Build history of the part. All positions in model axes, mm. Face numbers are marked on the shaded views. A direction names the side the tool comes from. Round coordinates to 2 decimals unless told otherwise and drop trailing zeros. Write each loop counter-clockwise with the first axis right and the second up, starting at its lowest first coordinate (ties: lowest second). Pieces come first, ordered by that corner, then holes.
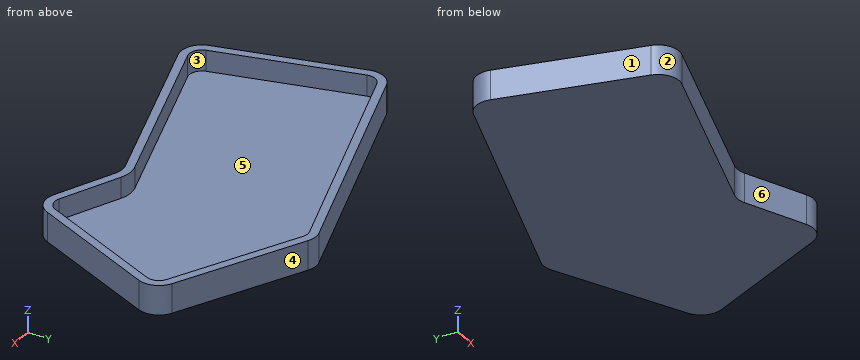
from build123d import *

# Parameters (mm, degrees)
F1_DEPTH = 20
F2_DEPTH = 50
F3_T     = -20


with BuildPart() as f1:
    # F0 (on Top) → F1 (new body)
    with BuildSketch(Plane.XY):
        with BuildLine():
            Line((126.4149565512, 318.7475000366), (-450.1034598535, 122.5814987763))
            ThreePointArc((-450.1034598535, 122.5814987763), (-478.0910883888, 98.8207080739), (-482.3054199281, 62.3498712928))
            Line((-482.3054199281, 62.3498712928), (-393.9558391633, -268.5866574495))
            ThreePointArc((-393.9558391633, -268.5866574495), (-369.4207710673, -299.6767597656), (-329.9698834283, -303.1683916176))
            Line((-329.9698834283, -303.1683916176), (106.3450430495, -159.0930914556))
            ThreePointArc((106.3450430495, -159.0930914556), (124.3346881302, -156.625037143), (142.0194350117, -160.7443028487))
            Line((142.0194350117, -160.7443028487), (282.7517397768, -222.1523142062))
            ThreePointArc((282.7517397768, -222.1523142062), (320.9333231451, -222.9008478399), (348.5065336168, -196.4790448091))
            Line((348.5065336168, -196.4790448091), (481.7955905074, 106.1445162961))
            ThreePointArc((481.7955905074, 106.1445162961), (483.0336988414, 143.3672853444), (458.1969646809, 171.1198362923))
            Line((458.1969646809, 171.1198362923), (164.6807282631, 316.2339391714))
            ThreePointArc((164.6807282631, 316.2339391714), (145.7983966372, 321.3050895289), (126.4149565512, 318.7475000366))
        make_face()
    extrude(amount=F1_DEPTH)

    # F2 (add): a face of the model
    f2_faces = [f1.faces().sort_by_distance(p)[0] for p in [
        (-7.672903893, 13.4350398808, 20),
    ]]
    extrude(f2_faces, amount=F2_DEPTH)

    # F3
    f3_openings = [f1.faces().sort_by_distance(p)[0] for p in [
        (-7.672904, 13.43504, 70),
    ]]
    offset(amount=F3_T, openings=f3_openings)


solid = f1.part
1) Wall check: L1, parallel to Z at x = -269, y = -80; L2, parallel to Y at x = -291, z = 51; L3, parallel to Y at x = -307, z = 46. Give the ranges that are in metal, low to high.
Results:
L1: z = 0 to 20
L2: y = -290.3 to -269.24, 155.59 to 176.72
L3: y = -295.58 to -274.52, 150.15 to 171.27
2) Slice it at D-D (y = 18). Write the cut outline in (x, z).
Results:
outline: (-470.47, 0) - (442.97, 0) - (442.97, 70) - (421.12, 70) - (421.12, 20) - (-449.76, 20) - (-449.76, 70) - (-470.47, 70) - close
3) Slice it at B-B (y = -172). Write the cut outline in (x, z), plus the area to 3 significant figures.
Results:
outline: (-419.74, 0) - (67.26, 0) - (67.26, 70) - (3.47, 70) - (3.47, 20) - (-399.04, 20) - (-399.04, 70) - (-419.74, 70) - close; (167.81, 0) - (359.29, 0) - (359.29, 70) - (337.43, 70) - (337.43, 20) - (217.82, 20) - (217.82, 70) - (167.81, 70) - close
area: 21,400 mm2
4) Which spindle directions (+Z, -Z, +X, -X, +Y, -Y) get a long thin tool onto all of the face, cutting with end or side? Do the marked faces 4, 5 and 6. Say none if no direction does.
Results:
face 4: +Z, -Z, +X, +Y
face 5: +Z
face 6: +Z, -Z, -Y
5) Slice it at C-C (x = 400). Write the cut outline in (y, z), plus the area to 3 significant figures.
Results:
outline: (-79.57, 0) - (199.89, 0) - (199.89, 70) - (177.58, 70) - (177.58, 20) - (-29.95, 20) - (-29.95, 70) - (-79.57, 70) - close
area: 9,190 mm2
6) Pin check, flat tips, straight feed: pin 1 Ø2 at (y, z) = (156, 16.5) entering from +X; pin 2 Ø12 at (x, z) = (-138.5, 17) entering from -Y; pin 3 Ø12 at (x, z) = (20.5, 50) entering from +Y. Stop position of each tip, or through.
Results:
pin 1: stops at x = 476.98
pin 2: stops at y = -241.92
pin 3: stops at y = 284.75
7) Mould opens along X. For the marked faces 1, 2 and 3 say: released by +X, released by -X, zero draft, split by the parting line, or undercut.
Results:
face 1: released by -X
face 2: split by the parting line
face 3: undercut
8) Slice it at A-A (z = 44). Write the cut outline in (x, y), plus the area to 3 significant figures.
Results:
outline: (-482.31, 62.35) - (-393.96, -268.59) arc R50 ccw to (-329.97, -303.17) - (106.35, -159.09) arc R50 cw to (142.02, -160.74) - (282.75, -222.15) arc R50 ccw to (348.51, -196.48) - (481.8, 106.14) arc R50 ccw to (458.2, 171.12) - (164.68, 316.23) arc R50 ccw to (126.41, 318.75) - (-450.1, 122.58) arc R50 ccw to start; hole (-462.98, 67.51) - (-374.63, -263.43) arc R30 ccw to (-336.24, -284.18) - (100.07, -140.1) arc R70 cw to (150.02, -142.41) - (290.75, -203.82) arc R30 ccw to (330.2, -188.42) - (463.49, 114.21) arc R30 ccw to (449.33, 153.19) - (155.82, 298.31) arc R30 ccw to (132.86, 299.81) - (-443.66, 103.65) arc R30 ccw to start
area: 50,900 mm2
